Autodesk Inventor part; units mm, degrees
ref_plane "YZ Plane" through (0, 0, 0) normal (1, 0, 0) x (0, 1, 0)
ref_plane "XZ Plane" through (0, 0, 0) normal (0, 1, 0) x (-1, 0, 0)
ref_plane "XY Plane" through (0, 0, 0) normal (0, 0, 1) x (1, 0, 0)
sketch "Sketch1" plane through (0, 0, 0) normal (0, 0, 1) x (1, 0, 0)
  line L0 (-2.54, -8.19) -> (2.54, -8.19)
  line L1 (2.54, -8.19) -> (2.54, 8.19)
  line L2 (-2.54, 8.19) -> (-2.54, -8.19)
  line L3 (-2.54, -8.19) -> (2.54, 8.19) construction
  line L4 (2.54, -8.19) -> (-2.54, 8.19) construction
  circle A0 centre (0, 16.6545) radius 2.5 construction
  circle A1 centre (0, 16.6545) radius 5
  arc A2 (6.8029, 15.0051) -> (-6.8044, 15.0114) centre (0, 16.6545) ccw
  line L5 (-2.54, 8.19) -> (-2.54, 10.2591)
  line L6 (2.54, 8.19) -> (2.54, 10.2869)
  line L7 (0, 0) -> (0, 10.7842) construction
  line L8 (-2.54, 10.2591) -> (-3.9944, 10.2511)
  line L9 (2.54, 10.2869) -> (3.9944, 10.2948)
  line L10 (-3.9944, 10.2511) -> (-4.1214, 3.9003)
  line L11 (3.9944, 10.2948) -> (4.1214, 3.9454)
  line L12 (-4.1214, 3.9003) -> (-6.8044, 15.0114)
  line L13 (4.1214, 3.9454) -> (6.8029, 15.0051)
  line L14 (0, 0) -> (0, 22.9511) construction
  point P0 (-3.2672, 10.2551)
  dimension "d2" = 5
  dimension "d3" = 10
  dimension "d4" = 14
  dimension "d8" = 1.5815
  dimension "d9" = 1.5815
  dimension "d10" = 6.35
  dimension "d11" = 6.35
  dimension "d18" = 1.4545
  dimension "d19" = 1.4545
  dimension "d31" = 2.54
  dimension "d32" = 2.54
  dimension "d33" = 0
extrude "Plate1" add sketch "Sketch1" along normal blind 1.5748
sketch "Sketch2" plane through (0, 0, 0) normal (0, 0, -1) x (-1, 0, 0)
  circle A0 centre (0, 16.6545) radius 5
  line L0 (-3.9944, 10.2948) -> (-4.1214, 3.9454)
  line L1 (-2.54, 10.2869) -> (-3.9944, 10.2948)
  line L2 (-2.54, -8.19) -> (-2.54, 10.2869)
  line L3 (2.54, -8.19) -> (-2.54, -8.19)
  line L4 (2.54, 10.2591) -> (2.54, -8.19)
  line L5 (3.9944, 10.2511) -> (2.54, 10.2591)
  line L6 (4.1214, 3.9003) -> (3.9944, 10.2511)
  line L7 (6.8044, 15.0114) -> (4.1214, 3.9003)
  arc A1 (6.8044, 15.0114) -> (-6.8029, 15.0051) centre (0, 16.6545) ccw
  line L8 (-4.1214, 3.9454) -> (-6.8029, 15.0051)
  line L9 (-1.5875, -17.19) -> (1.5875, -17.19)
  line L10 (1.5875, -17.19) -> (1.5875, 0.81)
  line L11 (1.5875, 0.81) -> (-1.5875, 0.81)
  line L12 (-1.5875, 0.81) -> (-1.5875, -17.19)
  line L13 (-1.5875, -17.19) -> (1.5875, 0.81) construction
  line L14 (1.5875, -17.19) -> (-1.5875, 0.81) construction
  point P0 (0, 0)
  point P1 (0, -8.19)
  dimension "d14" = 3.175
extrude "Extrusion1" cut sketch "Sketch2" against normal blind 25.4 contours L12 L11 L10 L3 | L3 L10 L9 L12
sketch "Sketch3" plane through (0, 0, 1.5748) normal (0, 0, 1) x (1, 0, 0)
  circle A0 centre (-37.757, 0) radius 3
  line L0 (-39.3445, -2.5456) -> (-36.1695, -2.5456)
  line L1 (-36.1695, -2.5456) -> (-36.1695, 2.5456)
  line L2 (-36.1695, 2.5456) -> (-39.3445, 2.5456)
  line L3 (-39.3445, 2.5456) -> (-39.3445, -2.5456)
  line L4 (-39.3445, -2.5456) -> (-36.1695, 2.5456) construction
  line L5 (-36.1695, -2.5456) -> (-39.3445, 2.5456) construction
  circle A1 centre (-37.757, 0) radius 4
  point P0 (0, 0)
  point P1 (-37.757, 3)
  point P2 (-37.757, 4)
  dimension "d35" = 8
  dimension "d28" = 6
  dimension "d29" = 3.175
  dimension "d30" = 5.0911
  dimension "d34" = 0.4545
  dimension "d36" = 1.4545
fillet "Fillet4" radius 0.381 6 edges at (-4.1214, 3.9003, 0.7874) (4.1214, 3.9454, 0.7874) (-2.54, -8.19, 0.7874) (-1.5875, -8.19, 0.7874) (1.5875, -8.19, 0.7874) (2.54, -8.19, 0.7874)
sketch "Sketch4" plane through (0, 0, 1.5748) normal (0, 0, 1) x (1, 0, 0)
  arc A0 (2.159, -8.19) -> (2.54, -7.809) centre (2.159, -7.809) ccw
  line L0 (2.54, 10.2869) -> (2.54, -7.809)
  line L1 (3.9944, 10.2948) -> (2.54, 10.2869)
  line L2 (4.0627, 6.8835) -> (3.9944, 10.2948)
  arc A1 (4.0627, 6.8835) -> (4.8139, 6.8013) centre (4.4436, 6.8911) ccw
  line L3 (6.8029, 15.0051) -> (4.8139, 6.8013)
  arc A2 (6.8029, 15.0051) -> (-6.8044, 15.0114) centre (0, 16.6545) ccw
  line L4 (-4.8137, 6.7674) -> (-6.8044, 15.0114)
  arc A3 (-4.8137, 6.7674) -> (-4.0625, 6.8492) centre (-4.4434, 6.8568) ccw
  line L5 (-3.9944, 10.2511) -> (-4.0625, 6.8492)
  line L6 (-2.54, 10.2591) -> (-3.9944, 10.2511)
  line L7 (-2.54, -7.809) -> (-2.54, 10.2591)
  arc A4 (-2.54, -7.809) -> (-2.159, -8.19) centre (-2.159, -7.809) ccw
  line L8 (-1.9685, -8.19) -> (-2.159, -8.19)
  arc A5 (-1.9685, -8.19) -> (-1.5875, -7.809) centre (-1.9685, -7.809) ccw
  line L9 (-1.5875, -7.809) -> (-1.5875, 0.81)
  line L10 (-1.5875, 0.81) -> (1.5875, 0.81)
  line L11 (1.5875, 0.81) -> (1.5875, -7.809)
  arc A6 (1.5875, -7.809) -> (1.9685, -8.19) centre (1.9685, -7.809) ccw
  line L12 (2.159, -8.19) -> (1.9685, -8.19)
  circle A7 centre (0, 16.6545) radius 5
  point P0 (0, 0)
extrude "Extrusion2" add sketch "Sketch4" against normal up to surface (1.5748 mm away) contours A7
sketch "Sketch5" plane through (0, 0, 1.5748) normal (0, 0, 1) x (1, 0, 0)
  arc A0 (2.159, -8.19) -> (2.54, -7.809) centre (2.159, -7.809) ccw
  line L0 (2.54, 10.2869) -> (2.54, -7.809)
  line L1 (3.9944, 10.2948) -> (2.54, 10.2869)
  line L2 (4.0627, 6.8835) -> (3.9944, 10.2948)
  arc A1 (4.0627, 6.8835) -> (4.8139, 6.8013) centre (4.4436, 6.8911) ccw
  line L3 (6.8029, 15.0051) -> (4.8139, 6.8013)
  arc A2 (6.8029, 15.0051) -> (-6.8044, 15.0114) centre (0, 16.6545) ccw
  line L4 (-4.8137, 6.7674) -> (-6.8044, 15.0114)
  arc A3 (-4.8137, 6.7674) -> (-4.0625, 6.8492) centre (-4.4434, 6.8568) ccw
  line L5 (-3.9944, 10.2511) -> (-4.0625, 6.8492)
  line L6 (-2.54, 10.2591) -> (-3.9944, 10.2511)
  line L7 (-2.54, -7.809) -> (-2.54, 10.2591)
  arc A4 (-2.54, -7.809) -> (-2.159, -8.19) centre (-2.159, -7.809) ccw
  line L8 (-1.9685, -8.19) -> (-2.159, -8.19)
  arc A5 (-1.9685, -8.19) -> (-1.5875, -7.809) centre (-1.9685, -7.809) ccw
  line L9 (-1.5875, -7.809) -> (-1.5875, 0.81)
  line L10 (-1.5875, 0.81) -> (1.5875, 0.81)
  line L11 (1.5875, 0.81) -> (1.5875, -7.809)
  arc A6 (1.5875, -7.809) -> (1.9685, -8.19) centre (1.9685, -7.809) ccw
  line L12 (2.159, -8.19) -> (1.9685, -8.19)
  arc A7 (1.5644, 14.7045) -> (-1.5644, 14.7045) centre (0, 16.6545) ccw
  line L13 (1.5644, 14.7045) -> (-1.5644, 14.7045)
  point P0 (0, 0)
  point P1 (0, 19.1545)
  dimension "d40" = 5
  dimension "d44" = 4.45
extrude "Extrusion3" cut sketch "Sketch5" against normal blind 25.4 contours L13 A7
chamfer "Chamfer3" distance 0.127 distance2 3.175 1 edges at (-2.54, 10.2591, 0.7874) measured on face at (-3.5096, 10.2538, 0.5249)
chamfer "Chamfer4" distance 3.175 distance2 0.127 1 edges at (2.54, 10.2869, 0.7874) measured on face at (2.54, -1.7771, 1.0499)
equation "\"d18\" = d36"
equation "\"d19\" = d36"
equation "\"BendRadius\" = Thickness"
equation "\"BendReliefWidth\" = Thickness"
equation "\"BendReliefDepth\" = 0.5 * Thickness"
equation "\"CornerReliefSize\" = 4 * Thickness"
equation "\"MinimumRemnant\" = 2 * Thickness"
equation "\"TransitionRadius\" = BendRadius"
equation "\"JacobiRadiusSize\" = BendRadius"
equation "\"GapSize\" = Thickness"
equation "\"d12\" = BendRadius"
properties part number "8mm OD 6mm ID Rod End125Motor"
Build history of the part. All positions in model axes, mm. A direction names the side the tool comes from. Coordinates: 2 decimals unless noted, no trailing zeros. Order: outer loops, then holes, each group sorted by start corner. A loop starts at its lowest first (then second) coordinate and runs counter-clockwise, first axis right, second up. Notation, with made-up numbers: (1, 21.5) - (8, 21.5) arc R16 cw to (8, 32.5) - close; hole circle Ø5 at (-22, 12.25). An arc over 180 degrees is marked (long way). Write each question's results on one line, items separated by ' | '. Start each with the question number.
Item 1: Band-saw the part on C-C on z = 1. Write the cut outline in (x, y), and give its area (3 significant figures).
Item 2: Band-saw the part on A-A on y = -6. Write the cut outline in (x, z).
Item 3: Mould opens along X. For faces 1 (the face through (-0.174, 23.652, 0.776)), 2 (the face through (-5.795, 10.832, 0.776)), 3 (the face through (1.588, -3, 1)) say: released by +X, released by -X, zero draft, split by the parting line, or undercut.
Item 4: Flat gauge pin, fed straight in: pin 1 (0.5 mm diameter, centred on y = -2.5, z = 1, fed in from -X). Where does the tip first touch, or does it go through?
Item 5: Band-saw the part on D-D on y = 9. Write the cut outline in (x, z).
Item 6: Band-saw the part on B-B on x = 0. Write the cut outline in (y, z), and give its area (3 significant figures).
Item 7: Wall check: probe 1 along Y at (x, z) = (0, 1.2); probe 2 along X at (y, z) = (3.5, 1.15); probe 3 along X at (y, z) = (0.5, 0.9). Give the ranges that are in metal, low to high. Write a range as [from, to].
Item 8: Tool access for faces 4 (the face through (-1.588, -4, 1)), 5 (the face through (5.794, 10.846, 0.776)), 6 (the face through (0, 14.704, 1)): list every direction of +Z, -Z, +X, -X, +Y, -Y with a clear straight run to the whole face (end or side of a thin tool).
Numbers:
1) outline: (-6.8, 15.01) - (-4.81, 6.77) arc R0.38 ccw to (-4.06, 6.85) - (-3.99, 10.25) - (-2.67, 10.26) - (-2.54, 7.08) - (-2.54, -7.81) arc R0.38 ccw to (-2.16, -8.19) - (-1.97, -8.19) arc R0.38 ccw to (-1.59, -7.81) - (-1.59, 0.81) - (1.59, 0.81) - (1.59, -7.81) arc R0.38 ccw to (1.97, -8.19) - (2.16, -8.19) arc R0.38 ccw to (2.54, -7.81) - (2.54, 7.11) - (2.67, 10.29) - (3.99, 10.29) - (4.06, 6.88) arc R0.38 ccw to (4.81, 6.8) - (6.8, 15.01) arc R7 ccw (long way) to start; hole (-1.56, 14.7) - (1.56, 14.7) arc R2.5 ccw (long way) to start | area: 215 mm^2
2) outline: (-2.54, 0) - (-1.59, 0) - (-1.59, 1.57) - (-2.54, 1.57) - close; (1.59, 0) - (2.54, 0) - (2.54, 1.57) - (1.59, 1.57) - close
3) face 1: split by the parting line | face 2: released by -X | face 3: undercut
4) pin 1: x = -2.54
5) outline: (-5.35, 0) - (-4.02, 0) - (-4.02, 1.57) - (-5.35, 1.57) - close; (-2.62, 0) - (2.62, 0) - (2.62, 1.57) - (-2.62, 1.57) - close; (4.02, 0) - (5.35, 0) - (5.35, 1.57) - (4.02, 1.57) - close
6) outline: (0.81, 0) - (14.7, 0) - (14.7, 1.57) - (0.81, 1.57) - close; (19.15, 0) - (23.65, 0) - (23.65, 1.57) - (19.15, 1.57) - close | area: 29.0 mm^2
7) probe 1: [0.81, 14.7], [19.15, 23.65] | probe 2: [-2.54, 2.54] | probe 3: [-2.54, -1.59], [1.59, 2.54]
8) face 4: +Z, -Z, -Y | face 5: +Z, -Z, +X, -Y | face 6: +Z, -Z
